Check sheet for the modelled part. Datum: model origin and axes. Units: mm. A direction names the side the tool comes from. Coordinates: 2 decimals unless noted, no trailing zeros. Write each question's results on one line, items separated by ' | '.
from build123d import *

# Parameters (mm, degrees)
F0_R     = 3.175
F1_DEPTH = 38.1
F2_W     = 25.4
F2_H     = 6.35
F3_DEPTH = 38.1
F4_R     = 6.35
F5_DEPTH = 1.5875
F5_TAPER = 60
F6_R     = 3.600369343
F7_DEPTH = 4.7635
F8_R     = 6.35
F9_R     = 1.5875


with BuildPart() as f1:
    # F0 (on Right) → F1 (new body)
    with BuildSketch(Plane.YZ):
        with BuildLine():
            Line((12.7, -3.175), (12.7, 3.175))
            Line((12.7, 3.175), (-8.0514773719, 3.175))
            ThreePointArc((-8.0514773719, 3.175), (-11.2264773719, 4.025738686), (-13.550738686, 6.35))
            ThreePointArc((-13.550738686, 6.35), (-24.549261314, 6.35), (-19.05, -3.175))
            Line((-19.05, -3.175), (12.7, -3.175))
        make_face()
        with Locations((-19.05, 3.175)):
            Circle(F0_R, mode=Mode.SUBTRACT)
    extrude(amount=F1_DEPTH)

    # F2 (on Right) → F3 (join)
    with BuildSketch(Plane.YZ):
        Rectangle(F2_W, F2_H)
    extrude(amount=-F3_DEPTH)

    # F4 (on face) → F5 (cut)
    with BuildSketch(Plane.XY.offset(3.175)):
        with Locations((19.05, 0)):
            Circle(F4_R)
        with Locations((-19.05, 0)):
            Circle(F4_R)
    extrude(amount=-F5_DEPTH, taper=F5_TAPER, mode=Mode.SUBTRACT)

    # F6 (on face) → F7 (cut, through all)
    with BuildSketch(Plane.XY.offset(1.5875)):
        with Locations((19.05, 0)):
            Circle(F6_R)
        with Locations((-19.05, 0)):
            Circle(F6_R)
    extrude(amount=-F7_DEPTH, mode=Mode.SUBTRACT)

    # F8
    f8_edges = [f1.edges().sort_by_distance(p)[0] for p in [
        (38.1, 12.7, 0),
        (-38.1, 12.7, 0),
        (-38.1, -12.7, 0),
    ]]
    fillet(f8_edges, radius=F8_R)

    # F9
    f9_edges = [f1.edges().sort_by_distance(p)[0] for p in [
        (0, 12.7, 3.175),
        (36.240128, 10.840128, 3.175),
    ]]
    fillet(f9_edges, radius=F9_R)


solid = f1.part
1. Go/stop test with flat-tipped pins: pin 1 (5 mm diameter, centred on x = 23, z = 6.5, fed in from +Y); pin 2 (2.5 mm diameter, centred on x = -14.5, z = 0.5, fed in from -Y); pin 3 (2 mm diameter, centred on x = 12, z = 3.5, fed in from +Y). Record where each tip stops, or that it passes through.
Values follow:
pin 1: stops at y = -11.18 | pin 2: stops at y = -12.7 | pin 3: stops at y = 12.41
2. Sectioned sample at A-A (x = 19.05). Give the number of separate pieces and of enclosed holes in the cut face, then the cut area to 3 significant figures.
Values follow:
separate pieces: 2 | enclosed holes: 1 | area: 217 mm^2
3. Draft check along Y on faces 4 (the cylindrical face through (-36.19, -10.89, 0.02)), 5 (the cylindrical face through (-22.647, 0.158, -0.76)), 6 (the cylindrical face through (-36.29, 10.79, 0.02)). Enter one of: pulls with the +Y half, pulls with the -Y half, needs draft (parallel to the pull), parting line crosses it, or undercut.
Values follow:
face 4: pulls with the -Y half | face 5: undercut | face 6: pulls with the +Y half
4. Access from +Z, -Z, +X, -X, +Y, -Y to the whole of each face (thin tool, end or side, straight path). Record for faces 1 (the cylindrical face through (37.623, -0.75, 2.722)), 2 (the cylindrical face through (-16.097, -12.223, -2.722)), 3 (the cylindrical face through (-15.653, -12.223, 2.722)).
Values follow:
face 1: +Z, +X, +Y | face 2: -Z, -X, -Y | face 3: +Z, -X, -Y
5. Material ranges on L1, parallel to Z at x = 11.5, y = -19.05 (3 decimals); L2, parallel to Z at x = -11, y = -6 (3 decimals); L3, parallel to X at y = 0.5, z = 0.75, recorded low to high. Write a range as [from, to].
Values follow:
L1: z = [-3.175, 0], [6.35, 9.525] | L2: z = [-3.175, 3.175] | L3: x = [-38.1, -22.62], [-15.48, 15.48], [22.62, 38.1]
